CAD build for the part. Positions are in the model's coordinates, mm. A direction names the side the tool comes from. Round coordinates to 2 decimals unless told otherwise and drop trailing zeros. Write each loop counter-clockwise with the first axis right and the second up, starting at its lowest first coordinate (ties: lowest second). Pieces come first, ordered by that corner, then holes. Notation, with made-up numbers: (-15, 57.5) - (0, 57.5) arc R7 cw to (0, 65.5) - close; hole circle Ø4 at (45, 37.25). An arc over 180 degrees is marked (long way). Answer in a Markdown table with one row per item.
```python
from build123d import *

# Parameters (mm, degrees)
F0_W     = 194.187328
F0_H     = 152.607068
F1_DEPTH = 93.218
F2_W     = 178.14736
F2_H     = 131.446124
F3_DEPTH = 149.606
F4_W     = 68.994268
F4_H     = 84.95936
F5_DEPTH = 236.728
F6_R     = 10.114418
F7_DEPTH = 293.624


with BuildPart() as f1:
    # F0 (on Top) → F1 (new body)
    with BuildSketch(Plane.XY):
        Rectangle(F0_W, F0_H)
    extrude(amount=F1_DEPTH)

    # F2 (on face) → F3 (cut)
    with BuildSketch(Plane.XY.offset(93.218)):
        Rectangle(F2_W, F2_H)
    extrude(amount=-F3_DEPTH, mode=Mode.SUBTRACT)

    # F4 (on face) → F5 (cut)
    with BuildSketch(Plane.XZ.offset(76.303534)):
        with Locations((0, 93.218)):
            Rectangle(F4_W, F4_H)
    extrude(amount=-F5_DEPTH, mode=Mode.SUBTRACT)

    # F6 (on face) → F7 (cut)
    with BuildSketch(Plane.YZ.offset(97.093664)):
        with Locations((0, 46.609)):
            Circle(F6_R)
    extrude(amount=-F7_DEPTH, mode=Mode.SUBTRACT)


solid = f1.part
```
Q1. Saw through at A-A on z = 66.5. List the corners of the cut face in (x, y).
Computed:
| item | result |
|---|---|
| outline | (-97.09, -76.3) - (-34.5, -76.3) - (-34.5, -65.72) - (-89.07, -65.72) - (-89.07, 65.72) - (-34.5, 65.72) - (-34.5, 76.3) - (-97.09, 76.3) - close; (34.5, -76.3) - (97.09, -76.3) - (97.09, 76.3) - (34.5, 76.3) - (34.5, 65.72) - (89.07, 65.72) - (89.07, -65.72) - (34.5, -65.72) - close |
Q2. Drill centre lines: line 1 (Y direction, x = -81, z = 87.5); line 2 (X direction, y = 44, z = 32.5); line 3 (Z direction, x = 91, y = 0). Where is each one in solid material? Low to high.
Computed:
| item | result |
|---|---|
| line 1 | y = -76.3 to -65.72, 65.72 to 76.3 |
| line 2 | x = -97.09 to -89.07, 89.07 to 97.09 |
| line 3 | z = 0 to 36.49, 56.72 to 93.22 |
Q3. Saw through at D-D on z = 29.5. List the corners of the cut face in (x, y).
Computed:
| item | result |
|---|---|
| outline | (-97.09, -76.3) - (97.09, -76.3) - (97.09, 76.3) - (-97.09, 76.3) - close; hole (-89.07, -65.72) - (89.07, -65.72) - (89.07, 65.72) - (-89.07, 65.72) - close |
Q4. Flat gauge pins, fed straight in: pin 1 (16 mm diameter, centred on y = 0, z = 46.609, fed in from -X); pin 2 (8.5 mm diameter, centred on x = 15, y = -73.5, fed in from +Z). Where does each tip first touch, or does it go through?
Computed:
| item | result |
|---|---|
| pin 1 | passes through |
| pin 2 | stops at z = 50.74 |
Q5. Saw through at C-C on y = 0. List the corners of the cut face in (x, z).
Computed:
| item | result |
|---|---|
| outline | (-97.09, 0) - (-89.07, 0) - (-89.07, 36.49) - (-97.09, 36.49) - close; (-97.09, 56.72) - (-89.07, 56.72) - (-89.07, 93.22) - (-97.09, 93.22) - close; (89.07, 0) - (97.09, 0) - (97.09, 36.49) - (89.07, 36.49) - close; (89.07, 56.72) - (97.09, 56.72) - (97.09, 93.22) - (89.07, 93.22) - close |
Q6. Saw through at B-B on x = 78. List the corners of the cut face in (y, z).
Computed:
| item | result |
|---|---|
| outline | (-76.3, 0) - (-65.72, 0) - (-65.72, 93.22) - (-76.3, 93.22) - close; (65.72, 0) - (76.3, 0) - (76.3, 93.22) - (65.72, 93.22) - close |
Q7. 3-axis set-ups, long thin cutter, end or side, ignore diameter. For faces 1 (the cylindrical face through (93.14, -2.193, 36.735)), 2 (the flat face through (-34.497, 71, 72)), 3 (the flat face through (-1, 65.723, 47)): which of +Z, -Z, +X, -X, +Y, -Y reach the whole face in a straight line?
Computed:
| item | result |
|---|---|
| face 1 | +X, -X |
| face 2 | +Z, +Y, -Y |
| face 3 | +Z, -Z |
Q8. Pull direction Y, two halves, no side cores. Call faces 4 (the flat face through (-1, 76.304, 46)), 5 (the flat face through (89.074, -1, 58)), 6 (the flat face through (34.497, 71, 72)): released by +Y, released by -Y, zero draft, split by the parting line, or undercut.
Computed:
| item | result |
|---|---|
| face 4 | released by +Y |
| face 5 | undercut |
| face 6 | zero draft |
